from build123d import *

# Parameters (mm, degrees)
F1_DEPTH = 3.175


with BuildPart() as f1:
    # F0 (on Right) → F1 (new body)
    with BuildSketch(Plane.YZ):
        with BuildLine():
            ThreePointArc((-419.804555, 263.773604), (-491.646604, 234.015653), (-521.404555, 162.173604))
            Line((-521.404555, 162.173604), (-521.404555, -414.946396))
            Line((-521.404555, -414.946396), (485.999445, -414.946396))
            Line((485.999445, -414.946396), (485.999445, 162.173604))
            ThreePointArc((485.999445, 162.173604), (456.241494, 234.015653), (384.399445, 263.773604))
            Line((384.399445, 263.773604), (-17.702555, 263.773604))
            Line((-17.702555, 263.773604), (-419.804555, 263.773604))
        make_face()
        with BuildLine():
            ThreePointArc((-419.804548, 69.353524), (-416.084804, 78.33378), (-407.104548, 82.053524))
            Line((-407.104548, 82.053524), (-381.704548, 82.053524))
            ThreePointArc((-381.704548, 82.053524), (-372.724292, 78.33378), (-369.004548, 69.353524))
            Line((-369.004548, 69.353524), (-369.004548, -355.246476))
            ThreePointArc((-369.004548, -355.246476), (-372.724292, -364.226732), (-381.704548, -367.946476))
            Line((-381.704548, -367.946476), (-407.104548, -367.946476))
            ThreePointArc((-407.104548, -367.946476), (-416.084804, -364.226732), (-419.804548, -355.246476))
            Line((-419.804548, -355.246476), (-419.804548, 69.353524))
        make_face(mode=Mode.SUBTRACT)
        with BuildLine():
            Line((-311.304543, -355.246476), (-311.304543, 69.353524))
            ThreePointArc((-311.304543, 69.353524), (-307.584799, 78.33378), (-298.604543, 82.053524))
            Line((-298.604543, 82.053524), (-273.204543, 82.053524))
            ThreePointArc((-273.204543, 82.053524), (-264.224287, 78.33378), (-260.504543, 69.353524))
            Line((-260.504543, 69.353524), (-260.504543, -355.246476))
            ThreePointArc((-260.504543, -355.246476), (-264.224287, -364.226732), (-273.204543, -367.946476))
            Line((-273.204543, -367.946476), (-298.604543, -367.946476))
            ThreePointArc((-298.604543, -367.946476), (-307.584799, -364.226732), (-311.304543, -355.246476))
        make_face(mode=Mode.SUBTRACT)
        with BuildLine():
            Line((-202.804543, -355.246476), (-202.804543, 69.353524))
            ThreePointArc((-202.804543, 69.353524), (-199.084799, 78.33378), (-190.104543, 82.053524))
            Line((-190.104543, 82.053524), (-164.704543, 82.053524))
            ThreePointArc((-164.704543, 82.053524), (-155.724287, 78.33378), (-152.004543, 69.353524))
            Line((-152.004543, 69.353524), (-152.004543, -355.246476))
            ThreePointArc((-152.004543, -355.246476), (-155.724287, -364.226732), (-164.704543, -367.946476))
            Line((-164.704543, -367.946476), (-190.104543, -367.946476))
            ThreePointArc((-190.104543, -367.946476), (-199.084799, -364.226732), (-202.804543, -355.246476))
        make_face(mode=Mode.SUBTRACT)
        with BuildLine():
            Line((-94.304543, -355.246476), (-94.304543, 69.353524))
            ThreePointArc((-94.304543, 69.353524), (-90.584799, 78.33378), (-81.604543, 82.053524))
            Line((-81.604543, 82.053524), (-56.204543, 82.053524))
            ThreePointArc((-56.204543, 82.053524), (-47.224287, 78.33378), (-43.504543, 69.353524))
            Line((-43.504543, 69.353524), (-43.504543, -355.246476))
            ThreePointArc((-43.504543, -355.246476), (-47.224287, -364.226732), (-56.204543, -367.946476))
            Line((-56.204543, -367.946476), (-81.604543, -367.946476))
            ThreePointArc((-81.604543, -367.946476), (-90.584799, -364.226732), (-94.304543, -355.246476))
        make_face(mode=Mode.SUBTRACT)
        with BuildLine():
            Line((14.195457, -355.246476), (14.195457, 69.353524))
            ThreePointArc((14.195457, 69.353524), (17.915201, 78.33378), (26.895457, 82.053524))
            Line((26.895457, 82.053524), (52.295457, 82.053524))
            ThreePointArc((52.295457, 82.053524), (61.275713, 78.33378), (64.995457, 69.353524))
            Line((64.995457, 69.353524), (64.995457, -355.246476))
            ThreePointArc((64.995457, -355.246476), (61.275713, -364.226732), (52.295457, -367.946476))
            Line((52.295457, -367.946476), (26.895457, -367.946476))
            ThreePointArc((26.895457, -367.946476), (17.915201, -364.226732), (14.195457, -355.246476))
        make_face(mode=Mode.SUBTRACT)
        with BuildLine():
            Line((122.695457, -355.246476), (122.695457, 69.353524))
            ThreePointArc((122.695457, 69.353524), (126.415201, 78.33378), (135.395457, 82.053524))
            Line((135.395457, 82.053524), (160.795457, 82.053524))
            ThreePointArc((160.795457, 82.053524), (169.775713, 78.33378), (173.495457, 69.353524))
            Line((173.495457, 69.353524), (173.495457, -355.246476))
            ThreePointArc((173.495457, -355.246476), (169.775713, -364.226732), (160.795457, -367.946476))
            Line((160.795457, -367.946476), (135.395457, -367.946476))
            ThreePointArc((135.395457, -367.946476), (126.415201, -364.226732), (122.695457, -355.246476))
        make_face(mode=Mode.SUBTRACT)
        with BuildLine():
            Line((231.195457, -355.246476), (231.195457, 69.353524))
            ThreePointArc((231.195457, 69.353524), (234.915201, 78.33378), (243.895457, 82.053524))
            Line((243.895457, 82.053524), (269.295457, 82.053524))
            ThreePointArc((269.295457, 82.053524), (278.275713, 78.33378), (281.995457, 69.353524))
            Line((281.995457, 69.353524), (281.995457, -355.246476))
            ThreePointArc((281.995457, -355.246476), (278.275713, -364.226732), (269.295457, -367.946476))
            Line((269.295457, -367.946476), (243.895457, -367.946476))
            ThreePointArc((243.895457, -367.946476), (234.915201, -364.226732), (231.195457, -355.246476))
        make_face(mode=Mode.SUBTRACT)
        with BuildLine():
            Line((339.695457, -355.246476), (339.695457, 69.353524))
            ThreePointArc((339.695457, 69.353524), (343.415201, 78.33378), (352.395457, 82.053524))
            Line((352.395457, 82.053524), (377.795457, 82.053524))
            ThreePointArc((377.795457, 82.053524), (386.775713, 78.33378), (390.495457, 69.353524))
            Line((390.495457, 69.353524), (390.495457, -355.246476))
            ThreePointArc((390.495457, -355.246476), (386.775713, -364.226732), (377.795457, -367.946476))
            Line((377.795457, -367.946476), (352.395457, -367.946476))
            ThreePointArc((352.395457, -367.946476), (343.415201, -364.226732), (339.695457, -355.246476))
        make_face(mode=Mode.SUBTRACT)
        with BuildLine():
            ThreePointArc((-419.804553, 200.273602), (-416.08481, 209.253859), (-407.104553, 212.973604))
            Line((-407.104553, 212.973604), (-381.704548, 212.973604))
            ThreePointArc((-381.704548, 212.973604), (-372.724292, 209.25386), (-369.004548, 200.273604))
            Line((-369.004548, 200.273604), (-369.004548, 178.048524))
            ThreePointArc((-369.004548, 178.048524), (-372.724292, 169.068268), (-381.704548, 165.348524))
            Line((-381.704548, 165.348524), (-407.10455, 165.348524))
            ThreePointArc((-407.10455, 165.348524), (-416.084805, 169.068267), (-419.80455, 178.048522))
            Line((-419.80455, 178.048522), (-419.804553, 200.273602))
        make_face(mode=Mode.SUBTRACT)
        with BuildLine():
            ThreePointArc((-298.604543, 165.348524), (-307.584799, 169.068268), (-311.304543, 178.048524))
            Line((-311.304543, 178.048524), (-311.304543, 200.273604))
            ThreePointArc((-311.304543, 200.273604), (-307.584799, 209.25386), (-298.604543, 212.973604))
            Line((-298.604543, 212.973604), (-273.204543, 212.973604))
            ThreePointArc((-273.204543, 212.973604), (-264.224287, 209.25386), (-260.504543, 200.273604))
            Line((-260.504543, 200.273604), (-260.504543, 178.048524))
            ThreePointArc((-260.504543, 178.048524), (-264.224287, 169.068268), (-273.204543, 165.348524))
            Line((-273.204543, 165.348524), (-298.604543, 165.348524))
        make_face(mode=Mode.SUBTRACT)
        with BuildLine():
            Line((-201.827555, 241.548524), (-17.702555, 241.548524))
            Line((-17.702555, 241.548524), (166.422445, 241.548524))
            ThreePointArc((166.422445, 241.548524), (175.402701, 237.82878), (179.122445, 228.848524))
            Line((179.122445, 228.848524), (179.122445, 178.048524))
            ThreePointArc((179.122445, 178.048524), (175.402701, 169.068268), (166.422445, 165.348524))
            Line((166.422445, 165.348524), (-201.827555, 165.348524))
            ThreePointArc((-201.827555, 165.348524), (-210.807811, 169.068268), (-214.527555, 178.048524))
            Line((-214.527555, 178.048524), (-214.527555, 228.848524))
            ThreePointArc((-214.527555, 228.848524), (-210.807811, 237.82878), (-201.827555, 241.548524))
        make_face(mode=Mode.SUBTRACT)
        with BuildLine():
            ThreePointArc((243.895457, 165.348524), (234.915201, 169.068268), (231.195457, 178.048524))
            Line((231.195457, 178.048524), (231.195457, 200.273604))
            ThreePointArc((231.195457, 200.273604), (234.915201, 209.25386), (243.895457, 212.973604))
            Line((243.895457, 212.973604), (269.295457, 212.973604))
            ThreePointArc((269.295457, 212.973604), (278.275713, 209.25386), (281.995457, 200.273604))
            Line((281.995457, 200.273604), (281.995457, 178.048524))
            ThreePointArc((281.995457, 178.048524), (278.275713, 169.068268), (269.295457, 165.348524))
            Line((269.295457, 165.348524), (243.895457, 165.348524))
        make_face(mode=Mode.SUBTRACT)
        with BuildLine():
            ThreePointArc((352.395457, 165.348524), (343.415201, 169.068268), (339.695457, 178.048524))
            Line((339.695457, 178.048524), (339.695457, 200.273604))
            ThreePointArc((339.695457, 200.273604), (343.415201, 209.25386), (352.395457, 212.973604))
            Line((352.395457, 212.973604), (377.795457, 212.973604))
            ThreePointArc((377.795457, 212.973604), (386.775713, 209.25386), (390.495457, 200.273604))
            Line((390.495457, 200.273604), (390.495457, 178.048524))
            ThreePointArc((390.495457, 178.048524), (386.775713, 169.068268), (377.795457, 165.348524))
            Line((377.795457, 165.348524), (352.395457, 165.348524))
        make_face(mode=Mode.SUBTRACT)
    extrude(amount=F1_DEPTH)


solid = f1.part
Input: part model. Units: mm. Frame: model coordinates. Round coordinates to 2 decimals unless told otherwise and drop trailing zeros. Answer as a JSON object with one key per item and string values. Group by question number.
1) Pin query (flat end, axial travel): pin 1 (1.6 mm diameter, centred on x = 2, z = 214.5, fed in from +Y); pin 2 (8 mm diameter, centred on y = 20.5, z = -263.5, fed in from +X); pin 3 (1.6 mm diameter, centred on x = 1.5, z = 190.5, fed in from -Y). Return the tip coordinate at first contact, or that it passes through.
2) Section query A-A on z = -250. State how many separate pieces and enclosed holes the cut face has, plus the area to 3 significant figures.
3) Ray query, L1, parallel to Z at x = 2.7, y = 34.5; L2, parallel to Z at x = 1.8, y = 358; L3, parallel to Z at x = 0.4, y = 70. Return the intervals inside material, ascending.
Reply:
{
 "1": {"pin 1": "stops at y = 471.96", "pin 2": "passes through", "pin 3": "stops at y = -517.6"},
 "2": {"separate pieces": "9", "enclosed holes": "0", "area": "1,910 mm2"},
 "3": {"L1": "z = -414.95 to -367.95, 82.05 to 165.35, 241.55 to 263.77", "L2": "z = -414.95 to -367.95, 82.05 to 165.35, 212.97 to 263.77", "L3": "z = -414.95 to 165.35, 241.55 to 263.77"}
}
